```python
from build123d import *

# Parameters (mm, degrees)
F0_R     = 1.5875
F1_DEPTH = 38.1
F2_R     = 3.3957745988
F3_DEPTH = 3.175
F4_DEPTH = 10.795


with BuildPart() as f1:
    # F0 (on Right) → F1 (new body)
    with BuildSketch(Plane.YZ):
        with Locations((-14.1914412379, 11.465549469)):
            Circle(F0_R)
    extrude(amount=F1_DEPTH)

    # F2 (on face) → F3 (join)
    with BuildSketch(Plane.YZ.offset(38.1)):
        with Locations((-14.1914412379, 11.465549469)):
            Circle(F2_R)
    extrude(amount=F3_DEPTH)

    # F4 (cut): a face of the model
    f4_faces = [f1.faces().sort_by_distance(p)[0] for p in [
        (0, -14.1914412379, 11.465549469),
    ]]
    extrude(f4_faces, amount=-F4_DEPTH, mode=Mode.SUBTRACT)


solid = f1.part
```
Build history of the part. All positions in model axes, mm. A direction names the side the tool comes from. Round coordinates to 2 decimals unless told otherwise and drop trailing zeros. Order: outer loops, then holes, each group sorted by start corner. A loop starts at its lowest first (then second) coordinate and runs counter-clockwise, first axis right, second up. Notation, with made-up numbers: (-11, -37) -> (41, -37) arc R37 cw to (41, 1) -> close; hole circle Ø10 at (-14.5, -6.75). An arc over 180 degrees is marked (long way). Answer in a Markdown table with one row per item.
1) Wall check: L1, parallel to X at y = -16.5, z = 9.5 (3 decimals); L2, parallel to Y at x = 14, z = 11.5; L3, parallel to Z at x = 14, y = -14.5. Give the ranges that are in metal, low to high.
Values:
| item | result |
|---|---|
| L1 | 38.1 to 41.275 |
| L2 | -15.78 to -12.6 |
| L3 | 9.91 to 13.02 |
2) Band-saw the part on C-C on x = 28.5. Give the cut face in (y, z) (1 decimal).
Values:
| item | result |
|---|---|
| outline | circle Ø3.2 at (-14.2, 11.5) |
3) Band-saw the part on A-A on y = -15. Give the cut face in (x, z) (3 decimals), and give its area (3 significant figures).
Values:
| item | result |
|---|---|
| outline | (10.795, 10.099) -> (38.1, 10.099) -> (38.1, 8.167) -> (41.275, 8.167) -> (41.275, 14.764) -> (38.1, 14.764) -> (38.1, 12.832) -> (10.795, 12.832) -> close |
| area | 95.5 mm2 |
4) Band-saw the part on D-D on y = -16.5. Give the cut face in (x, z) (3 decimals), and give its area (3 significant figures).
Values:
| item | result |
|---|---|
| outline | (38.1, 8.975) -> (41.275, 8.975) -> (41.275, 13.956) -> (38.1, 13.956) -> close |
| area | 15.8 mm2 |
5) Band-saw the part on B-B on z = 10.5. Give the cut face in (x, y) (3 decimals), and give its area (3 significant figures).
Values:
| item | result |
|---|---|
| outline | (10.795, -15.452) -> (38.1, -15.452) -> (38.1, -17.447) -> (41.275, -17.447) -> (41.275, -10.936) -> (38.1, -10.936) -> (38.1, -12.931) -> (10.795, -12.931) -> close |
| area | 89.5 mm2 |
6) Pin check, flat tips, straight feed: P1, Ø4, axis at x = 29, y = -14, coming from the +Z side; P2, Ø4, axis at x = 15, z = 13, coming from the +Y side; P3, Ø2, axis at x = 20.5, z = 11.5, coming from the -Y side. Stop position of each tip, or through.
Values:
| item | result |
|---|---|
| P1 | z = 13.05 |
| P2 | y = -12.6 |
| P3 | y = -15.78 |
7) Which spindle directions (+Z, -Z, +X, -X, +Y, -Y) get a long thin tool onto all of the face, cutting with end or side? Do faces 1 (the cylindrical face through (39.665, -16.694, 13.761)), 2 (the flat face through (38.1, -13, 10)). Say none if no direction does.
Values:
| item | result |
|---|---|
| face 1 | +X, -X |
| face 2 | -X |
